from build123d import *

# Parameters (mm, degrees)
F0_W     = 45
F0_H     = 70
F1_DEPTH = 3
F3_DEPTH = 10
F4_SIZE  = 9.99999


# Not quite as in the source:
# - a fillet or chamfer is up to 0.001 mm smaller than in the source, because OpenCascade refuses the exact size


with BuildPart() as f1:
    # F0 (on Top) → F1 (new body)
    with BuildSketch(Plane.XY):
        Rectangle(F0_W, F0_H)
    extrude(amount=F1_DEPTH)

    # F2 (on face) → F3 (join)
    with BuildSketch(Plane.XY.offset(3)):
        Polygon((-18.5, 20), (-18.5, 31), (-7.5, 31), (-7.5, 35), (-22.5, 35), (-22.5, 20), align=None)
        Polygon((7.5, 35), (7.5, 31), (18.5, 31), (18.5, 20), (22.5, 20), (22.5, 35), align=None)
        Polygon((18.5, -31), (7.5, -31), (7.5, -35), (22.5, -35), (22.5, -20), (18.5, -20), align=None)
        Polygon((-18.5, -31), (-18.5, -20), (-22.5, -20), (-22.5, -35), (-7.5, -35), (-7.5, -31), align=None)
    extrude(amount=F3_DEPTH)

    # F4 (size 10 in the source; OpenCascade refuses exactly that, so slightly less here)
    f4_edges = [f1.edges().sort_by_distance(p)[0] for p in [
        (-7.5, 33, 13),
        (-7.5, -33, 13),
        (-20.5, -20, 13),
        (20.5, -20, 13),
        (20.5, 20, 13),
        (-20.5, 20, 13),
        (7.5, -33, 13),
        (7.5, 33, 13),
    ]]
    chamfer(f4_edges, length=F4_SIZE)


solid = f1.part
Geometry check sheet. Reference: the model listing, model coordinates, mm. A direction names the side the tool comes from. Give positions to 0.01 mm unless a question says otherwise; leave off trailing zeros. Loops run counter-clockwise (first coordinate to the right, second up) from the corner with the lowest first, then second, coordinate; pieces in that order, holes last. Notation, with made-up numbers: (16.25, 70.5) -> (50.25, 70.5) arc R16 ccw to (50.25, 96.5) -> close; hole circle Ø9 at (30.5, 87). An arc over 180 degrees is marked (long way). Answer in a Markdown table with one row per item. Add a question column.
1) Cross-section at D-D on x = -10.5. Record the boundary of the cut face in (y, z), and give its area (3 significant figures).
2) Gauge pin test, flat ends, axial feed: P1, Ø2, axis at x = -9, y = -2, coming from the +Z side; P2, Ø3, axis at y = 25.5, z = 9.5, coming from the -X side; P3, Ø1, axis at x = 12.5, z = 11.5, coming from the -Y side. Record the tip position at first contact, or that the pin passes through.
3) Cross-section at C-C on y = -25. Record the boundary of the cut face in (x, z), and give its area (3 significant figures).
4) Draft check along Y on faces 4 (the face through (-22.5, 0, 2)), 5 (the face through (0, -35, 2)), 6 (the face through (21, -25, 8)). Enter one of: pulls with the +Y half, pulls with the -Y half, needs draft (parallel to the pull), parting line crosses it, or undercut.
5) Cross-section at B-B on z = 5.75. Record the boundary of the cut face in (x, y).
6) Material ranges on probe 1 along Y at (x, z) = (10, 4.5); probe 2 along Z at (x, y) = (-5, 30); probe 3 along X at (y, z) = (-27, 7), recorded low to high. Write a range as from..to.
7) Set-up check for faces 1 (the face through (-12.4, 33, 7.9)), 2 (the face through (18.5, 27, 7)), 3 (the face through (20, 25, 8)): record each of +Z, -Z, +X, -X, +Y, -Y from which the full face is reachable in a straight line by a thin tool's end or side.
Outcome:
| question | item | result |
|---|---|---|
| 1 | outline | (-35, 0) -> (35, 0) -> (35, 6) -> (31, 6) -> (31, 3) -> (-31, 3) -> (-31, 6) -> (-35, 6) -> close |
| 1 | area | 234 mm^2 |
| 2 | P1 | stops at z = 3 |
| 2 | P2 | stops at x = -22.5 |
| 2 | P3 | passes through |
| 3 | outline | (-22.5, 0) -> (22.5, 0) -> (22.5, 8) -> (18.5, 8) -> (18.5, 3) -> (-18.5, 3) -> (-18.5, 8) -> (-22.5, 8) -> close |
| 3 | area | 175 mm^2 |
| 4 | face 4 | needs draft |
| 4 | face 5 | pulls with the -Y half |
| 4 | face 6 | undercut |
| 5 | outline | (-22.5, -35) -> (-10.25, -35) -> (-10.25, -31) -> (-18.5, -31) -> (-18.5, -22.75) -> (-22.5, -22.75) -> close; (-22.5, 22.75) -> (-18.5, 22.75) -> (-18.5, 31) -> (-10.25, 31) -> (-10.25, 35) -> (-22.5, 35) -> close; (10.25, -35) -> (22.5, -35) -> (22.5, -22.75) -> (18.5, -22.75) -> (18.5, -31) -> (10.25, -31) -> close; (10.25, 31) -> (18.5, 31) -> (18.5, 22.75) -> (22.5, 22.75) -> (22.5, 35) -> (10.25, 35) -> close |
| 6 | probe 1 | y = -35..-31, 31..35 |
| 6 | probe 2 | z = 0..3 |
| 6 | probe 3 | x = -22.5..-18.5, 18.5..22.5 |
| 7 | face 1 | +Z, +Y, -Y |
| 7 | face 2 | +Z |
| 7 | face 3 | +Z, +X, -X |
